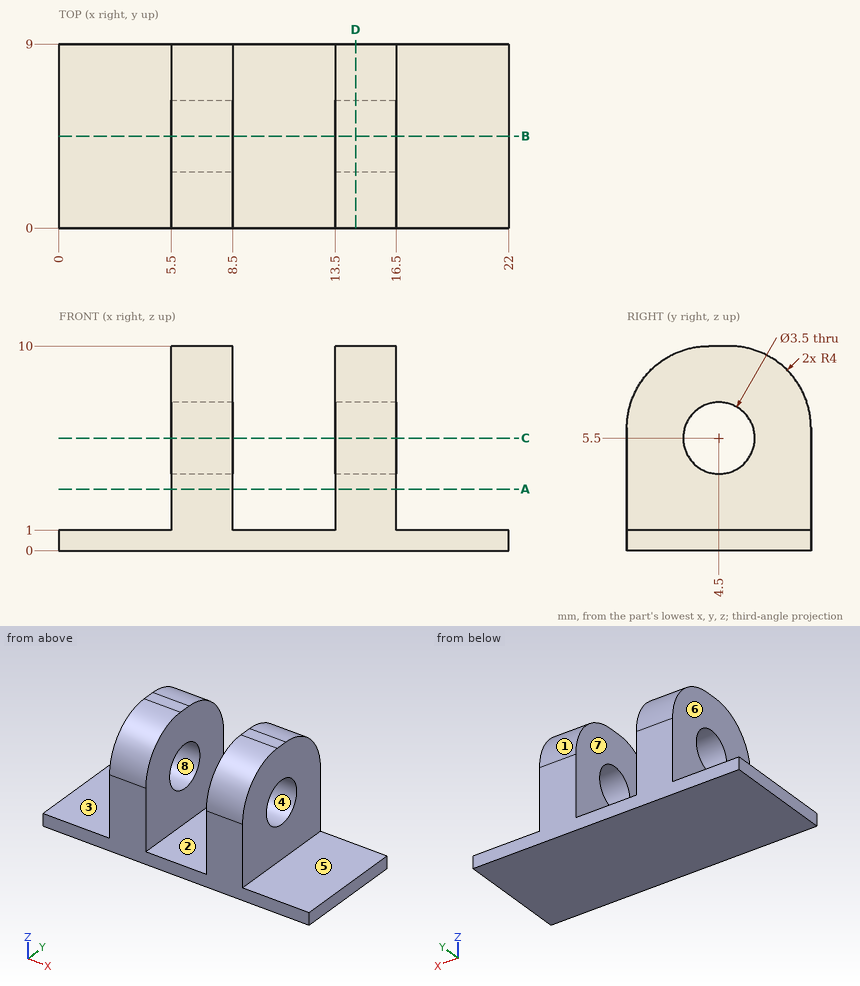
For this review, use the dimensioned drawing (mm, ordinates from the lowest corner) and the shaded views. A direction names the side the tool comes from. Round coordinates to 2 decimals unless told otherwise and drop trailing zeros. Write each loop counter-clockwise with the first axis right and the second up, starting at its lowest first coordinate (ties: lowest second). Pieces come first, ordered by that corner, then holes. Notation, with made-up numbers: M 15.5,17.25 L 51.5,17.25 A22 cw 51.5,51.25 Z; hole C -34,-24.5 d1. An arc over 180 degrees is marked long. Write item = value, one per line. Start each with the question number.
(1) We need section D-D (x = 14.5). Give the boundary of the cut face in (y, z).
(2) For line 1 along X through (y, z) = (2.5, 5.75); line 2 along Y through (x, z) = (14.75, 5.5); line 3 along Z through (x, y) = (7.5, 6), list the stretches that pass through material, from the lowest coordinate up.
(3) We need section C-C (z = 5.5). Give the boundary of the cut face in (x, y).
(4) We need section B-B (y = 4.5). Give the boundary of the cut face in (x, z).
(5) Clearance check with flat-ended pins moving along their axes: pin 1 Ø3 at (x, y) = (12.5, 6.5) entering from +Z; pin 2 Ø1.6 at (x, y) = (18.5, 6) entering from +Z; pin 3 Ø4.5 at (y, z) = (3, 3.5) entering from -X; pin 4 Ø4 at (x, z) = (12.5, 7) entering from +Y. State where each tip first meets the part, or that it passes through.
(6) We need section A-A (z = 3). Give the boundary of the cut face in (x, y), then the cut area to 3 significant figures.
(7) For the marked faces 1, 2, 3, 4 and 5, list the 3-axis set-ups (+Z, -Z, +X, -X, +Y, -Y) from which the entire face can be reached by the end or side of a thin tool; tool diameter is ignored.
(8) The part is to be moulded in two halves that separate along X. For the marked faces 6, 7 and 8, say which applies: +X half, -X half, draft (parallel to the pull), parting line (faces both ways), or undercut.
Results found:
q1.outline = M 0,0 L 9,0 L 9,6 A4 ccw 5,10 L 4,10 A4 ccw 0,6 Z; hole C 4.5,5.5 d3.5
q2.line_1 = 5.5 to 8.5, 13.5 to 16.5
q2.line_2 = 0 to 2.75, 6.25 to 9
q2.line_3 = 0 to 4.6, 6.4 to 9.87
q3.outline = M 5.5,0 L 8.5,0 L 8.5,2.75 L 5.5,2.75 Z; M 5.5,6.25 L 8.5,6.25 L 8.5,9 L 5.5,9 Z; M 13.5,0 L 16.5,0 L 16.5,2.75 L 13.5,2.75 Z; M 13.5,6.25 L 16.5,6.25 L 16.5,9 L 13.5,9 Z
q4.outline = M 0,0 L 22,0 L 22,1 L 16.5,1 L 16.5,3.75 L 13.5,3.75 L 13.5,1 L 8.5,1 L 8.5,3.75 L 5.5,3.75 L 5.5,1 L 0,1 Z; M 5.5,7.25 L 8.5,7.25 L 8.5,10 L 5.5,10 Z; M 13.5,7.25 L 16.5,7.25 L 16.5,10 L 13.5,10 Z
q5.pin_1 = 9.98
q5.pin_2 = 1
q5.pin_3 = 5.5
q5.pin_4 = 9
q6.outline = M 5.5,0 L 8.5,0 L 8.5,9 L 5.5,9 Z; M 13.5,0 L 16.5,0 L 16.5,9 L 13.5,9 Z
q6.area = 54.0 mm²
q7.face_1 = +Z, +X, -X, +Y
q7.face_2 = +Z, +Y, -Y
q7.face_3 = +Z, -X, +Y, -Y
q7.face_4 = +X, -X
q7.face_5 = +Z, +X, +Y, -Y
q8.face_6 = -X half
q8.face_7 = undercut
q8.face_8 = draft
